from build123d import *

# Parameters (mm, degrees)
SKETCH001_W          = 5
SKETCH001_H          = 1
POCKET_DEPTH         = 16.5
SKETCH002_R          = 55
SKETCH002_W          = 42.3
SKETCH002_H          = 42.3
POCKET001_DEPTH      = 0.001
POCKET001_DEPTH_BACK = -42.501
SKETCH003_R          = 1.75
POCKET002_DEPTH      = 5
SKETCH004_W          = 8
SKETCH004_H          = 8
PAD_DEPTH            = 5


with BuildPart() as part:
    # Sketch → Revolution (revolve)
    with BuildSketch(Plane.XZ):
        Polygon((0, 0), (26.9, 0), (26.9, 20.5), (10.9875, 20.5), (10.9875, 22.5), (2.497, 22.5), (2.497, 42.5), (0, 42.5), align=None)
    revolve(axis=Axis((0, 0, 0), (0, 0, 1)))

    # Sketch001 → Pocket (cut)
    with BuildSketch(Plane.XY.offset(42.5)):
        with Locations((0, 2.6)):
            Rectangle(SKETCH001_W, SKETCH001_H)
    extrude(amount=-POCKET_DEPTH, mode=Mode.SUBTRACT)

    # Sketch002 → Pocket001 (cut, two sides)
    with BuildSketch(Plane.XY) as pocket001_sk:
        Circle(SKETCH002_R)
        Rectangle(SKETCH002_W, SKETCH002_H, mode=Mode.SUBTRACT)
    extrude(amount=-POCKET001_DEPTH, mode=Mode.SUBTRACT)
    extrude(pocket001_sk.sketch, amount=-POCKET001_DEPTH_BACK, mode=Mode.SUBTRACT)

    # Sketch003 (on Face10 of Pocket001) → Pocket002 (cut)
    with BuildSketch(Plane(origin=(0, 0, 20.5), x_dir=(-1, 0, 0), z_dir=(0, 0, 1))):
        with Locations((-15.5, 15.5)):
            Circle(SKETCH003_R)
        with Locations((15.5, 15.5)):
            Circle(SKETCH003_R)
        with Locations((15.5, -15.5)):
            Circle(SKETCH003_R)
        with Locations((-15.5, -15.5)):
            Circle(SKETCH003_R)
    extrude(amount=-POCKET002_DEPTH, mode=Mode.SUBTRACT)

    # Sketch004 → Pad (join)
    with BuildSketch(Plane.XY.offset(2.3)):
        with Locations((0, -25.15)):
            Rectangle(SKETCH004_W, SKETCH004_H)
    extrude(amount=PAD_DEPTH)


solid = part.part
Can you work these out from the model? Positions are in its coordinate system, mm. A direction names the side the tool comes from. Give positions to 0.01 mm unless a question says otherwise; leave off trailing zeros. Loops run counter-clockwise (first coordinate to the right, second up) from the corner with the lowest first, then second, coordinate; pieces in that order, holes last. Notation, with made-up numbers: (16.25, 18.25) - (57.25, 18.25) arc R26 cw to (57.25, 50.25) - close; hole circle Ø9 at (-39, 43.25). An arc over 180 degrees is marked (long way). Return JSON: item names as keys, results as strings.
1. I want a section at A-A on z = 19. Please give me the cut outline in (x, y).
Output values:
{"outline": "(-21.15, -16.62) arc R26.9 ccw to (-16.62, -21.15) - (16.62, -21.15) arc R26.9 ccw to (21.15, -16.62) - (21.15, 16.62) arc R26.9 ccw to (16.62, 21.15) - (-16.62, 21.15) arc R26.9 ccw to (-21.15, 16.62) - close; hole circle Ø3.5 at (-15.5, -15.5); hole circle Ø3.5 at (-15.5, 15.5); hole circle Ø3.5 at (15.5, -15.5); hole circle Ø3.5 at (15.5, 15.5)"}
2. We'd pull the mould along Y, two halves only. Please class faces 6 (the face through (0, 21.15, 10)), 7 (the face through (-21.15, 0, 10)), 8 (the face through (16, -16, 15.5)): +Y half, -Y half, draft (parallel to the pull), parting line (faces both ways), or undercut.
Output values:
{"face 6": "+Y half", "face 7": "draft", "face 8": "undercut"}
3. I want a section at C-C on x = 15.5. Please give me the cut outline in (y, z).
Output values:
{"outline": "(-21.15, 0) - (21.15, 0) - (21.15, 20.5) - (17.25, 20.5) - (17.25, 15.5) - (13.75, 15.5) - (13.75, 20.5) - (-13.75, 20.5) - (-13.75, 15.5) - (-17.25, 15.5) - (-17.25, 20.5) - (-21.15, 20.5) - close"}
4. For faces 1 (the face through (4, -25, 5)), 2 (the face through (0, -25, 7.3)), 3 (the face through (-18.99, 19.05, 10.39)), 4 (the face through (-1.43, 10.894, 21.514)), 5 (the face through (-4, -25, 5)), which set-ups out of +Z, -Z, +X, -X, +Y, -Y let a thin tool reach every point of the face, with its end or its side?
Output values:
{"face 1": "+Z, -Z, +X, -Y", "face 2": "+Z, +X, -X, -Y", "face 3": "+Z, -Z, -X, +Y", "face 4": "+Z", "face 5": "+Z, -Z, -X, -Y"}
5. If I drill on line 1 (Y direction, x = 15.5, z = 18.2); line 2 (Z direction, x = -11, y = 7.5), over which ranges is the centre line in solid material (lowest first)?
Output values:
{"line 1": "y = -21.15 to -17.25, -13.75 to 13.75, 17.25 to 21.15", "line 2": "z = 0 to 20.5"}
6. I want a section at D-D on z = 14. Please give me the cut outline in (x, y).
Output values:
{"outline": "(-21.15, -16.62) arc R26.9 ccw to (-16.62, -21.15) - (16.62, -21.15) arc R26.9 ccw to (21.15, -16.62) - (21.15, 16.62) arc R26.9 ccw to (16.62, 21.15) - (-16.62, 21.15) arc R26.9 ccw to (-21.15, 16.62) - close"}
7. I want a section at B-B on y = 0. Please give me the cut outline in (x, z).
Output values:
{"outline": "(-21.15, 0) - (21.15, 0) - (21.15, 20.5) - (10.99, 20.5) - (10.99, 22.5) - (2.5, 22.5) - (2.5, 42.5) - (-2.5, 42.5) - (-2.5, 22.5) - (-10.99, 22.5) - (-10.99, 20.5) - (-21.15, 20.5) - close"}
8. I'm going to push flat-ended pins straight in: pin 1 Ø1.8 at (x, y) = (-15.5, 15) entering from +Z; pin 2 Ø3 at (x, y) = (15.5, -15) entering from +Z; pin 3 Ø12 at (x, z) = (-5.5, 35) entering from -Y. Where does each tip first touch, or does it pass through?
Output values:
{"pin 1": "stops at z = 15.5", "pin 2": "stops at z = 20.5", "pin 3": "stops at y = -2.5"}
